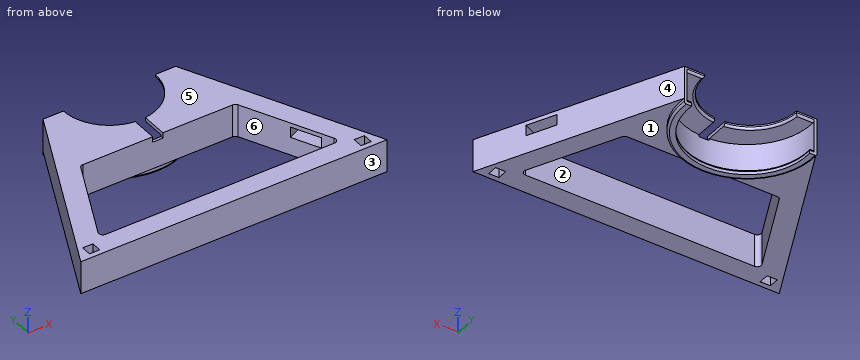
from build123d import *

# Parameters (mm, degrees)
BOSS_EXTRUDE1_DEPTH = 16
SKETCH2_R           = 31.25
CUT_EXTRUDE1_DEPTH  = 14.2
SKETCH3_R           = 22.5
CUT_EXTRUDE2_DEPTH  = 14.2
FILLET1_R           = 2
SKETCH4_W           = 5.2
SKETCH4_H           = 14.5
CUT_EXTRUDE3_DEPTH  = 10
SKETCH5_W           = 5
SKETCH5_H           = 5
CUT_EXTRUDE4_DEPTH  = 119.241278748
SKETCH6_W           = 5
SKETCH6_H           = 15
CUT_EXTRUDE5_DEPTH  = 2.7
BOSS_EXTRUDE2_DEPTH = 2.5
FILLET2_R           = 1
FILLET3_R           = 1


with BuildPart() as part:
    # Sketch1 → Boss-Extrude1 (new body)
    with BuildSketch(Plane.XY):
        Polygon((-75, 0), (75, 0), (32.5, 90), (-32.5, 90), align=None)
        Polygon((-59.218872646, 10), (-37.968872646, 55), (37.968872646, 55), (59.218872646, 10), align=None, mode=Mode.SUBTRACT)
    extrude(amount=BOSS_EXTRUDE1_DEPTH)

    # Sketch2 → Cut-Extrude1 (cut)
    with BuildSketch(Plane(origin=(0, 0, 0), x_dir=(-1, 0, 0), z_dir=(0, 0, -1))):
        with Locations((0, 87.5)):
            Circle(SKETCH2_R)
    extrude(amount=-CUT_EXTRUDE1_DEPTH, mode=Mode.SUBTRACT)

    # Sketch3 → Cut-Extrude2 (cut)
    with BuildSketch(Plane(origin=(0, 0, 14.2), x_dir=(-1, 0, 0), z_dir=(0, 0, -1))):
        with Locations((0, 90)):
            Circle(SKETCH3_R)
    extrude(amount=-CUT_EXTRUDE2_DEPTH, mode=Mode.SUBTRACT)

    # Fillet1
    fillet1_edges = [part.edges().sort_by_distance(p)[0] for p in [
        (59.218872646, 10, 8),
        (37.968872646, 55, 8),
        (-37.968872646, 55, 8),
        (-59.218872646, 10, 8),
    ]]
    fillet(fillet1_edges, radius=FILLET1_R)

    # Sketch4 → Cut-Extrude3 (cut)
    with BuildSketch(Plane(origin=(61.324921136, 28.958990536, 0), x_dir=(0, 0, -1), z_dir=(0.9042486467459909, 0.42700630540782925, 0))):
        with Locations((-11.4, 0.254673281)):
            Rectangle(SKETCH4_W, SKETCH4_H)
    extrude(amount=-CUT_EXTRUDE3_DEPTH, mode=Mode.SUBTRACT)

    # Sketch5 → Cut-Extrude4 (cut, through all)
    with BuildSketch(Plane(origin=(0, 0, 0), x_dir=(-1, 0, 0), z_dir=(0, 0, -1))):
        with Locations((-66.5, 5)):
            Rectangle(SKETCH5_W, SKETCH5_H)
        with Locations((66.5, 5)):
            Rectangle(SKETCH5_W, SKETCH5_H)
    extrude(amount=-CUT_EXTRUDE4_DEPTH, mode=Mode.SUBTRACT)

    # Sketch6 → Cut-Extrude5 (cut)
    with BuildSketch(Plane.XY.offset(16)):
        with Locations((0, 62.5)):
            Rectangle(SKETCH6_W, SKETCH6_H)
    extrude(amount=-CUT_EXTRUDE5_DEPTH, mode=Mode.SUBTRACT)

    # Sketch7 → Boss-Extrude2 (add)
    with BuildSketch(Plane(origin=(0, 0, 0), x_dir=(-1, 0, 0), z_dir=(0, 0, -1))):
        with BuildLine():
            Line((-32.5, 90), (-28.892040426, 90))
            ThreePointArc((-28.892040426, 90), (0, 58.5), (28.892040426, 90))
            Line((28.892040426, 90), (32.5, 90))
            ThreePointArc((32.5, 90), (0, 54.903987974), (-32.5, 90))
        make_face()
    extrude(amount=BOSS_EXTRUDE2_DEPTH)

    # Fillet2
    fillet2_edges = [part.edges().sort_by_distance(p)[0] for p in [
        (0, 54.903987974, -2.5),
    ]]
    fillet(fillet2_edges, radius=FILLET2_R)

    # Fillet3
    fillet3_edges = [part.edges().sort_by_distance(p)[0] for p in [
        (-16.770509831, 75, 14.2),
        (-30.020939956, 90, 0),
        (0, 58.5, 0),
        (30.020939956, 90, 0),
        (-26.824919743, 90, 14.2),
        (26.824919743, 90, 14.2),
        (16.770509831, 75, 14.2),
    ]]
    fillet(fillet3_edges, radius=FILLET3_R)


solid = part.part
Build history of the part. All positions in model axes, mm. Face numbers are marked on the shaded views. A direction names the side the tool comes from. Coordinates: 2 decimals unless noted, no trailing zeros. Order: outer loops, then holes, each group sorted by start corner. A loop starts at its lowest first (then second) coordinate and runs counter-clockwise, first axis right, second up. Notation, with made-up numbers: (-28.75, 9) - (19.25, 9) arc R19 cw to (19.25, 27) - close; hole circle Ø3 at (14.25, 12). An arc over 180 degrees is marked (long way). Write item = value, one per line. Start each with the question number.
1) Flat gauge pins, fed straight in: pin 1 Ø2 at (y, z) = (37, 6.5) entering from +X; pin 2 Ø5.5 at (y, z) = (6, 5) entering from -X; pin 3 Ø5 at (x, y) = (51.5, 22.5) entering from -Z; pin 4 Ø5 at (x, y) = (-44, 75.5) entering from -Z. Where does each tip first touch, or does it go through?
2) Saw through at A-A on x = 0. Write the cut outline in (y, z), then the cut area to 3 significant figures.
3) Saw through at C-C on z = 2.5. Write the cut outline in (x, y).
4) Saw through at B-B on y = 39.5. Write the cut outline in (x, z).
5) 3-axis set-ups, long thin cutter, end or side, ignore diameter. For the marked faces 1, 2 and 3: which of +Z, -Z, +X, -X, +Y, -Y reach the whole face in a straight line?
6) Wall check: line 1 along X through (y, z) = (87.5, -1.9); line 2 along X through (y, z) = (87.5, -1.5); line 3 along Z through (x, y) = (-13.5, 67). Give the ranges that are in metal, low to high. Write a range as from..to.
7) Two-plate mould, pull along Y, no slides. Class the marked faces 4, 5 and 6: pulls with the +Y half, pulls with the -Y half, needs draft (parallel to the pull), parting line crosses it, or undercut.
From the geometry:
q1.pin_1 = 58
q1.pin_2 = -73.47
q1.pin_3 = 0
q1.pin_4 = through
q2.outline = (0, 0) - (10, 0) - (10, 16) - (0, 16) - close; (54.9, -1.5) arc R1 ccw to (55.9, -2.5) - (58.5, -2.5) - (58.5, -1) arc R1 ccw to (57.5, 0) - (56.25, 0) - (56.25, 13.3) - (55, 13.3) - (55, 0) - (54.9, 0) - close
q2.area = 185 mm^2
q3.outline = (-75, 0) - (75, 0) - (32.5, 90) - (31.15, 90) arc R31.25 cw (long way) to (-31.15, 90) - (-32.5, 90) - close; hole (-69, 2.5) - (-64, 2.5) - (-64, 7.5) - (-69, 7.5) - close; hole (-57.87, 12.85) arc R2 ccw to (-56.06, 10) - (56.06, 10) arc R2 ccw to (57.87, 12.85) - (38.51, 53.85) arc R2 ccw to (36.7, 55) - (-36.7, 55) arc R2 ccw to (-38.51, 53.85) - close; hole (64, 2.5) - (69, 2.5) - (69, 7.5) - (64, 7.5) - close
q4.outline = (-56.35, 0) - (-45.29, 0) - (-45.29, 16) - (-56.35, 16) - close; (45.29, 0) - (56.35, 0) - (56.35, 16) - (45.29, 16) - close
q5.face_1 = -Z, -Y
q5.face_2 = +Z, -Z
q5.face_3 = +Z, -Z, +X, -X, -Y
q6.line_1 = -32.51..-29, 29..32.51
q6.line_2 = -32.6..-29, 29..32.6
q6.line_3 = 14.2..16
q7.face_4 = pulls with the +Y half
q7.face_5 = needs draft
q7.face_6 = undercut
